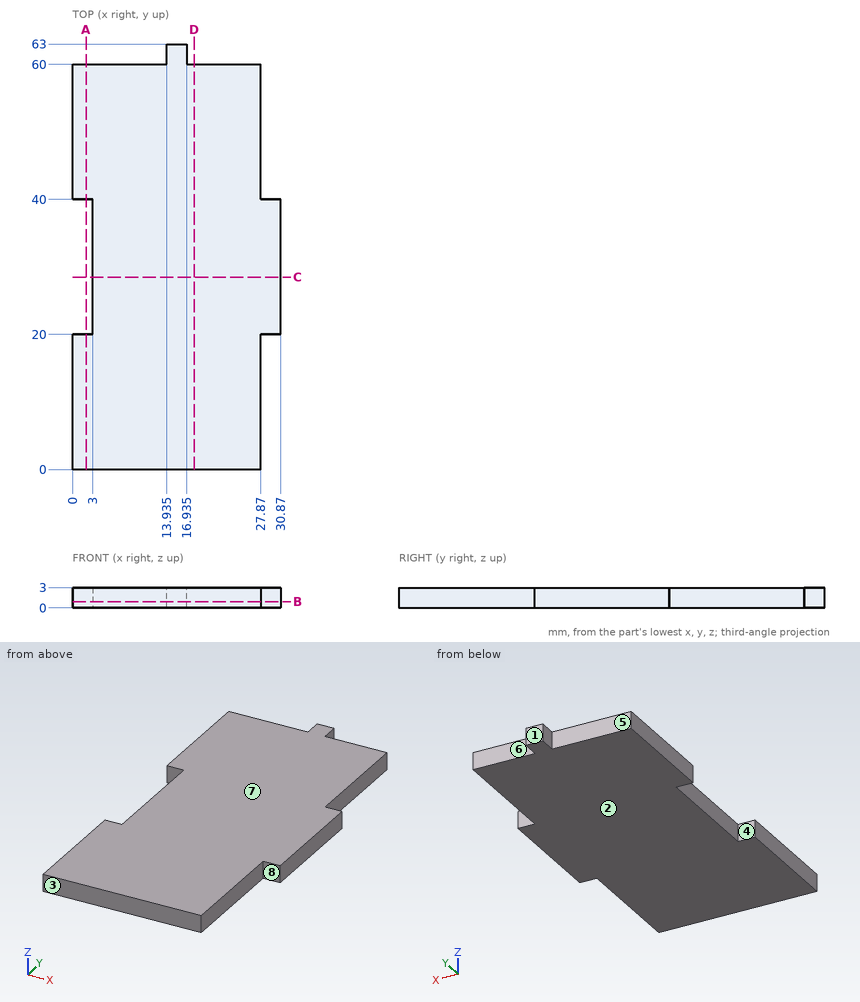
Here's the drawing with two shaded views (mm, measured from the low corner). I have some questions. A direction names the side the tool comes from. Round coordinates to 2 decimals unless told otherwise and drop trailing zeros. Loops run counter-clockwise (first coordinate to the right, second up) from the corner with the lowest first, then second, coordinate; pieces in that order, holes last. Notation, with made-up numbers: (-33, 19) - (-8, 19) arc R27 ccw to (-8, 54) - close; hole circle Ø6 at (26.25, 68). An arc over 180 degrees is marked (long way). Use CSV: the item, a comma, the result in double quotes. Start each with the question number.
1) For pin 1 Ø0.9 at (y, z) = (6.5, 1) entering from +X; pin 2 Ø0.9 at (x, z) = (30, 1) entering from -Y; pin 3 Ø1.5 at (y, z) = (26.5, 1) entering from -X, each with a flat end and sliding along its axis, tell me the tip position at first contact or that it passes through.
2) If we section it at D-D on x = 18: Write out the boundary of the cut face in (y, z), plus the area to 3 significant figures.
3) We'd pull the mould along Y, two halves only. Please class the marked faces 1, 2, 3 and 4: released by +Y, released by -Y, zero draft, split by the parting line, or undercut.
4) If we section it at A-A on x = 2: Write out the boundary of the cut face in (y, z), plus the area to 3 significant figures.
5) If we section it at B-B on z = 0.9: Write out the boundary of the cut face in (x, y) (3 decimals).
6) For the marked faces 5, 6, 7 and 8, which set-ups out of +Z, -Z, +X, -X, +Y, -Y let a thin tool reach every point of the face, with its end or its side?
7) If we section it at C-C on y = 28.5: Write out the boundary of the cut face in (x, z).
8) Please list where these lines run through material, in increasing order: probe 1 along Y at (x, z) = (19, 1.25); probe 2 along X at (y, z) = (42, 0.6); probe 3 along X at (y, z) = (38, 1.4). Write a range as [from, to].
Geometry results:
1,pin 1,"stops at x = 27.87"
1,pin 2,"stops at y = 20"
1,pin 3,"stops at x = 3"
2,outline,"(0, 0) - (60, 0) - (60, 3) - (0, 3) - close"
2,area,"180 mm2"
3,face 1,"released by +Y"
3,face 2,"zero draft"
3,face 3,"released by -Y"
3,face 4,"undercut"
4,outline,"(0, 0) - (20, 0) - (20, 3) - (0, 3) - close; (40, 0) - (60, 0) - (60, 3) - (40, 3) - close"
4,area,"120 mm2"
5,outline,"(0, 0) - (27.87, 0) - (27.87, 20) - (30.87, 20) - (30.87, 40) - (27.87, 40) - (27.87, 60) - (16.935, 60) - (16.935, 63) - (13.935, 63) - (13.935, 60) - (0, 60) - (0, 40) - (3, 40) - (3, 20) - (0, 20) - close"
6,face 5,"+Z, -Z, -X, +Y"
6,face 6,"+Z, -Z, +X, +Y"
6,face 7,"+Z, +X, -X, +Y, -Y"
6,face 8,"+Z, -Z, +X, -Y"
7,outline,"(3, 0) - (30.87, 0) - (30.87, 3) - (3, 3) - close"
8,probe 1,"y = [0, 60]"
8,probe 2,"x = [0, 27.87]"
8,probe 3,"x = [3, 30.87]"
